The listing builds one solid part. Answer for the finished solid, in the listing's coordinates (mm). Give positions to 0.01 mm unless a question says otherwise; leave off trailing zeros. Loops run counter-clockwise (first coordinate to the right, second up) from the corner with the lowest first, then second, coordinate; pieces in that order, holes last. Notation, with made-up numbers: (82.25, 73.5) - (94.25, 73.5) arc R21 cw to (94.25, 107.5) - close; hole circle Ø7 at (70.25, -33). An arc over 180 degrees is marked (long way). Write item = value, one per line. Start each with the question number.
1) The part is cut by section C-C on y = 81.25. Write down the section's boundary in (x, z).
2) The part is cut by section D-D on z = 3. Write down the section's boundary in (x, y), plus the area to 3 significant figures.
3) The part is cut by section A-A on x = -219.2. State how many separate pieces and enclosed holes the cut face has, plus the area to 3 significant figures.
4) The part is cut by section B-B on z = 5.75. Write down the section's boundary in (x, y), plus the area to 3 significant figures.
5) Consider probe 1 along Y at (x, z) = (-219.3, 2.75); probe 2 along Y at (x, z) = (-219.35, 6.5); probe 3 along Y at (x, z) = (-219.1, 5). Determine where each line is inside the solid, lowest interval first.
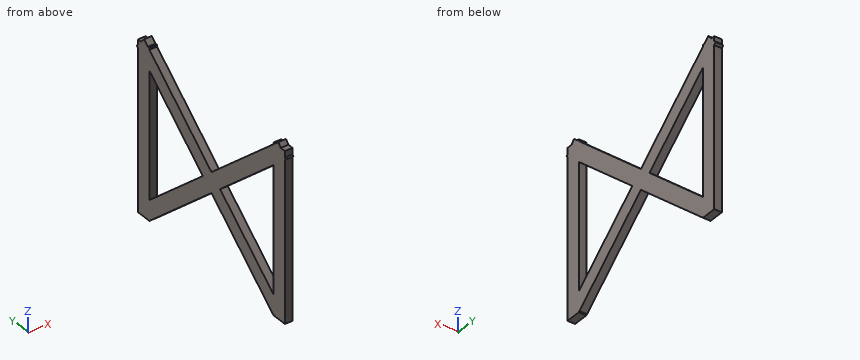
from build123d import *

# Parameters (mm, degrees)
BOX208_W          = 0.5
BOX208_H          = 1
BOX208_DEPTH      = 11
BOX209_W          = 0.5
BOX209_H          = 1
BOX209_DEPTH      = 16
BOX209_ROLL_ANGLE = 49
BOX210_W          = 0.5
BOX210_H          = 1
BOX210_DEPTH      = 16
BOX210_ROLL_ANGLE = -49
BOX207_W          = 0.5
BOX207_H          = 1
BOX207_DEPTH      = 11


with BuildPart() as cubo208:
    # Box208 → Box208 (new body)
    with BuildSketch(Plane(origin=(0, 12, 0.5), x_dir=(1, 0, 0), z_dir=(0, 0, 1))):
        with Locations((0.25, 0.5)):
            Rectangle(BOX208_W, BOX208_H)
    extrude(amount=BOX208_DEPTH)


with BuildPart() as cubo209:
    # Box209 → Box209 (new body)
    with BuildSketch(Plane.XY):
        with Locations((0.25, 0.5)):
            Rectangle(BOX209_W, BOX209_H)
    extrude(amount=BOX209_DEPTH)


with BuildPart() as cubo209_1:
    # Box209 roll: moved
    add(cubo209.part.rotate(Axis((0, 0, 0), (1, 0, 0)), BOX209_ROLL_ANGLE))


with BuildPart() as cubo209_2:
    # Box209 placement: moved
    add(cubo209_1.part.moved(Location((0, 12, 0.5))))


with BuildPart() as cubo210:
    # Box210 → Box210 (new body)
    with BuildSketch(Plane.XY):
        with Locations((0.25, 0.5)):
            Rectangle(BOX210_W, BOX210_H)
    extrude(amount=BOX210_DEPTH)


with BuildPart() as cubo210_1:
    # Box210 roll: moved
    add(cubo210.part.rotate(Axis((0, 0, 0), (1, 0, 0)), BOX210_ROLL_ANGLE))


with BuildPart() as cubo210_2:
    # Box210 placement: moved
    add(cubo210_1.part.moved(Location((0, 0.4, 1.3))))


with BuildPart() as fusion014:
    # Box207 → Box207 (new body)
    with BuildSketch(Plane.XY.offset(0.5)):
        with Locations((0.25, 0.5)):
            Rectangle(BOX207_W, BOX207_H)
    extrude(amount=BOX207_DEPTH)

    # Fusion014: union Cubo208, Cubo209, Cubo210
    add(cubo208.part)
    add(cubo209_2.part)
    add(cubo210_2.part)


with BuildPart() as fusion014_1:
    # Fusion014 placement: moved
    add(fusion014.part.moved(Location((-219.5, 70, 0))))


solid = fusion014_1.part
Answer below:
q1.outline = (-219.5, 1.15) - (-219, 1.15) - (-219, 2.48) - (-219.5, 2.48) - close; (-219.5, 9.41) - (-219, 9.41) - (-219, 10.73) - (-219.5, 10.73) - close
q2.outline = (-219.5, 70) - (-219, 70) - (-219, 71) - (-219.5, 71) - close; (-219.5, 72.36) - (-219, 72.36) - (-219, 73.88) - (-219.5, 73.88) - close; (-219.5, 79.12) - (-219, 79.12) - (-219, 80.65) - (-219.5, 80.65) - close; (-219.5, 82) - (-219, 82) - (-219, 83) - (-219.5, 83) - close
q2.area = 2.52 mm2
q3.separate_pieces = 1
q3.enclosed_holes = 2
q3.area = 50.3 mm2
q4.outline = (-219.5, 70) - (-219, 70) - (-219, 71) - (-219.5, 71) - close; (-219.5, 75.52) - (-219, 75.52) - (-219, 77.48) - (-219.5, 77.48) - close; (-219.5, 82) - (-219, 82) - (-219, 83) - (-219.5, 83) - close
q4.area = 1.98 mm2
q5.probe_1 = 70 to 71, 72.07 to 73.59, 79.41 to 80.94, 82 to 83
q5.probe_2 = 70 to 71, 75.1 to 77.91, 82 to 83
q5.probe_3 = 70 to 71, 74.66 to 76.18, 76.82 to 78.35, 82 to 83
